```python
from build123d import *

# Parameters (mm, degrees)
ESBO_O1_W                = 46.4
ESBO_O1_H                = 22
ESBO_O1_W_2              = 45
ESBO_O1_H_2              = 20.5
RESSALTO_EXTRUS_O1_DEPTH = 14
ESBO_O2_W                = 46.4
ESBO_O2_H                = 22
RESSALTO_EXTRUS_O2_DEPTH = 0.7
ESBO_O3_W                = 2.9
ESBO_O3_H                = 3.3
RESSALTO_EXTRUS_O3_DEPTH = 11
ESBO_O4_W                = 4.95750459
ESBO_O4_H                = 14
ESBO_O4_W_2              = 1
ESBO_O4_H_2              = 2.660947199
ESBO_O4_H_3              = 4
RESSALTO_EXTRUS_O4_DEPTH = 5
ESBO_O5_W                = 1
ESBO_O5_H                = 2.660947199
ESBO_O5_W_2              = 4.96
ESBO_O5_H_2              = 14
RESSALTO_EXTRUS_O5_DEPTH = 5
RESSALTO_EXTRUS_O9_DEPTH = 1
ESBO_O15_W               = 4.95750459
ESBO_O15_H               = 5
ESBO_O15_W_2             = 4.96
CORTE_EXTRUS_O3_DEPTH    = 2.5
ESBO_O16_R               = 0.95
CORTE_EXTRUS_O4_DEPTH    = 4
CORTE_EXTRUS_O7_DEPTH    = 11
CORTE_EXTRUS_O8_DEPTH    = 11
CORTE_EXTRUS_O9_START    = -4
ESBO_O20_R               = 0.95
CORTE_EXTRUS_O9_DEPTH    = 4


with BuildPart() as part:
    # Esboço1 → Ressalto-extrusão1 (new body)
    with BuildSketch(Plane(origin=(0, 0, 0), x_dir=(1, 0, 0), z_dir=(0, 1, 0))):
        Rectangle(ESBO_O1_W, ESBO_O1_H)
        Rectangle(ESBO_O1_W_2, ESBO_O1_H_2, mode=Mode.SUBTRACT)
    extrude(amount=RESSALTO_EXTRUS_O1_DEPTH)

    # Esboço2 → Ressalto-extrusão2 (add)
    with BuildSketch(Plane(origin=(0, 0, 0), x_dir=(1, 0, 0), z_dir=(0, 1, 0))):
        Rectangle(ESBO_O2_W, ESBO_O2_H)
    extrude(amount=-RESSALTO_EXTRUS_O2_DEPTH)

    # Esboço3 → Ressalto-extrusão3 (add)
    with BuildSketch(Plane(origin=(0, 0, 0), x_dir=(1, 0, 0), z_dir=(0, 1, 0))):
        with Locations((-14.05, 1.9)):
            Rectangle(ESBO_O3_W, ESBO_O3_H)
        with Locations((-14.05, 8.6)):
            Rectangle(ESBO_O3_W, ESBO_O3_H)
        with Locations((14.05, -8.6)):
            Rectangle(ESBO_O3_W, ESBO_O3_H)
        with Locations((14.05, -1.9)):
            Rectangle(ESBO_O3_W, ESBO_O3_H)
    extrude(amount=RESSALTO_EXTRUS_O3_DEPTH)

    # Esboço4 → Ressalto-extrusão4 (add)
    with BuildSketch(Plane.XY.offset(-10.25)):
        with Locations((-20.021247705, 7)):
            Rectangle(ESBO_O4_W, ESBO_O4_H)
        with Locations((-16, 1.3304736)):
            Rectangle(ESBO_O4_W_2, ESBO_O4_H_2)
        with Locations((-16, 12)):
            Rectangle(ESBO_O4_W_2, ESBO_O4_H_3)
    extrude(amount=RESSALTO_EXTRUS_O4_DEPTH)

    # Esboço5 → Ressalto-extrusão5 (add)
    with BuildSketch(Plane(origin=(0, 0, 10.25), x_dir=(-1, 0, 0), z_dir=(0, 0, -1))):
        Polygon((-15.5, 14), (-16.5, 14), (-16.5, 10), (-15.5, 10), (-15.5, 11), align=None)
        with Locations((-16, 1.3304736)):
            Rectangle(ESBO_O5_W, ESBO_O5_H)
        with Locations((-20.02, 7)):
            Rectangle(ESBO_O5_W_2, ESBO_O5_H_2)
    extrude(amount=RESSALTO_EXTRUS_O5_DEPTH)

    # Esboço10 → Ressalto-extrusão9 (add)
    with BuildSketch(Plane(origin=(0, 0, 0), x_dir=(1, 0, 0), z_dir=(0, 1, 0))):
        Polygon((15.5, 0.25), (-12.6, 0.25), (-12.6, 10.25), (22.5, 10.25), (22.5, -10.25), (15.5, -10.25), align=None)
    extrude(amount=RESSALTO_EXTRUS_O9_DEPTH)

    # Esboço15 → Corte-extrusão3 (cut, symmetric)
    with BuildSketch(Plane.XZ.offset(0.7)):
        with Locations((-20.021247705, -2.75)):
            Rectangle(ESBO_O15_W, ESBO_O15_H)
        with Locations((20.02, 2.75)):
            Rectangle(ESBO_O15_W_2, ESBO_O15_H)
    extrude(amount=CORTE_EXTRUS_O3_DEPTH, both=True, mode=Mode.SUBTRACT)

    # Esboço16 → Corte-extrusão4 (cut)
    with BuildSketch(Plane.XZ.offset(0.7)):
        with Locations(Location((-20.372, -8, 0), (0, 0, 270))):
            Circle(ESBO_O16_R)
        with Locations(Location((20.372, 8, 0), (0, 0, 270))):
            Circle(ESBO_O16_R)
    extrude(amount=-CORTE_EXTRUS_O4_DEPTH, mode=Mode.SUBTRACT)

    # Esboço18 → Corte-extrusão7 (cut)
    with BuildSketch(Plane.XY.offset(-0.25)):
        with BuildLine():
            Line((-10.6, 0.5), (-10.6, 1))
            Line((-10.6, 1), (-9.6, 1))
            Line((-9.6, 1), (-9.6, 0.5))
            ThreePointArc((-9.6, 0.5), (-10.1, 0), (-10.6, 0.5))
        make_face()
    extrude(amount=-CORTE_EXTRUS_O7_DEPTH, mode=Mode.SUBTRACT)

    # Esboço19 → Corte-extrusão8 (cut)
    with BuildSketch(Plane(origin=(0, 0, -11), x_dir=(-1, 0, 0), z_dir=(0, 0, -1))):
        with BuildLine():
            Line((-10.6, 0.5), (-10.6, 1))
            Line((-10.6, 1), (-9.6, 1))
            Line((-9.6, 1), (-9.6, 0.5))
            ThreePointArc((-9.6, 0.5), (-10.1, 0), (-10.6, 0.5))
        make_face()
    extrude(amount=-CORTE_EXTRUS_O8_DEPTH, mode=Mode.SUBTRACT)

    # Esboço20 → Corte-extrusão9 (cut)
    with BuildSketch(Plane(origin=(0, 14, 0), x_dir=(1, 0, 0), z_dir=(0, 1, 0)).offset(CORTE_EXTRUS_O9_START)):
        with Locations(Location((20.372, -8, 0), (0, 0, 90))):
            Circle(ESBO_O20_R)
        with Locations(Location((-20.372, 8, 0), (0, 0, 90))):
            Circle(ESBO_O20_R)
    extrude(amount=CORTE_EXTRUS_O9_DEPTH, mode=Mode.SUBTRACT)


solid = part.part
```
The model under review builds one solid part; all positions refer to its coordinate system, in mm. A direction names the side the tool comes from. Give positions to 0.01 mm unless a question says otherwise; leave off trailing zeros. Write each loop counter-clockwise with the first axis right and the second up, starting at its lowest first coordinate (ties: lowest second). Pieces come first, ordered by that corner, then holes.
(1) Tool access review of faces 3 (the flat face through (-1.8, 14, -10.5)), 4 (the flat face through (-15.5, 6, -9)), 5 (the flat face through (-12.6, 0.5, -5.2)): name each direction out of +Z, -Z, +X, -X, +Y, -Y from which nothing blocks a thin tool from reaching the whole face with its end or side.
(2) For P1, Ø0.9, axis at x = 13.5, z = 2, coming from the +Y side; P2, Ø1, axis at x = 2.5, z = 2, coming from the +Y side; P3, Ø5, axis at x = 0.5, z = 1, coming from the +Y side, all flat-tipped, find the tip position at first contact; note any pin that passes through.
(3) Consider section D-D, the plane x = -15. Give the boundary of the cut face in (y, z).
(4) The part is to be moulded in two halves that separate along Z. For faces 1 (the cylindrical face through (10.1, 0, -5.7)), 2 (the flat face through (15.5, 6, 9)), say which applies: released by +Z, released by -Z, zero draft, split by the parting line, or undercut.
(5) Consider section A-A, the plane z = 0.75. Give the boundary of the cut face in (x, y), and give its area (3 significant figures).
(6) To check wall thickness, follow L1, parallel to Z at x = 14, y = 0.5; L2, parallel to X at y = 3.25, z = -0.5; L3, parallel to X at y = 7, z = 3.25. State the ranges of each line that lie inside material, in increasing order.
(7) Consider section B-B, the plane y = 5.75. Give the boundary of the cut face in (x, z).
Returned:
1. face 3: +Z, -Z, +X, -X, +Y
1. face 4: none
1. face 5: +Y
2. P1: stops at y = 11
2. P2: stops at y = 0
2. P3: stops at y = 1
3. outline: (-0.7, -11) - (14, -11) - (14, -10.25) - (11, -10.25) - (11, -6.95) - (0, -6.95) - (0, -3.55) - (11, -3.55) - (11, -0.25) - (0, -0.25) - (0, 10.25) - (14, 10.25) - (14, 11) - (-0.7, 11) - close
4. face 1: zero draft
4. face 2: undercut
5. outline: (-23.2, -0.7) - (17.54, -0.7) - (17.54, 1) - (15.5, 1) - (15.5, 11) - (12.6, 11) - (12.6, 0) - (-22.5, 0) - (-22.5, 14) - (-23.2, 14) - close; (22.5, -0.7) - (23.2, -0.7) - (23.2, 14) - (22.5, 14) - close
5. area: 82.5 mm2
6. L1: z = -11 to -0.25, 0.25 to 3.55, 6.95 to 11
6. L2: x = -23.2 to -22.5, -15.5 to -12.6, 22.5 to 23.2
6. L3: x = -23.2 to -22.5, 12.6 to 15.5, 22.5 to 23.2
7. outline: (-23.2, -11) - (23.2, -11) - (23.2, 11) - (-23.2, 11) - close; (-15.5, -3.55) - (-12.6, -3.55) - (-12.6, -0.25) - (-15.5, -0.25) - close; (12.6, 0.25) - (15.5, 0.25) - (15.5, 3.55) - (12.6, 3.55) - close; hole (-22.5, -5.25) - (-17.54, -5.25) - (-17.54, -10.25) - (-15.5, -10.25) - (-15.5, -6.95) - (-12.6, -6.95) - (-12.6, -10.25) - (22.5, -10.25) - (22.5, 5.25) - (17.54, 5.25) - (17.54, 10.25) - (15.5, 10.25) - (15.5, 6.95) - (12.6, 6.95) - (12.6, 10.25) - (-22.5, 10.25) - close
